Can you work these out from the model? Positions are in its coordinate system, mm. A direction names the side the tool comes from. Round coordinates to 2 decimals unless told otherwise and drop trailing zeros. Order: outer loops, then holes, each group sorted by start corner. A loop starts at its lowest first (then second) coordinate and runs counter-clockwise, first axis right, second up. Notation, with made-up numbers: M 39,-8 L 93,-8 A29 ccw 93,26 Z; hole C -13,-9.5 d4. An arc over 180 degrees is marked long. One line per question, with ' | ' between items.
```python
from build123d import *

# Parameters (mm, degrees)
SKETCH1_R           = 27.62
BOSS_EXTRUDE1_DEPTH = 6
SKETCH2_R           = 16
SKETCH2_R_2         = 14
BOSS_EXTRUDE2_DEPTH = 36
CUT_EXTRUDE1_START  = -36
SKETCH3_R           = 14
CUT_EXTRUDE1_DEPTH  = 36
CHAMFER1_SIZE       = 5
CHAMFER1_SIZE2      = 7.140740034
CHAMFER2_SIZE       = 1
SKETCH4_R           = 27
SKETCH4_R_2         = 25
CUT_EXTRUDE2_DEPTH  = 1.6
FILLET1_R           = 2
FILLET2_R           = 4


with BuildPart() as part:
    # Sketch1 → Boss-Extrude1 (new body)
    with BuildSketch(Plane(origin=(0, 0, 0), x_dir=(1, 0, 0), z_dir=(0, 1, 0))):
        with Locations(Location((0, 0, 0), (0, 0, 270))):
            Circle(SKETCH1_R)
    extrude(amount=BOSS_EXTRUDE1_DEPTH)

    # Sketch2 → Boss-Extrude2 (add)
    with BuildSketch(Plane(origin=(0, 6, 0), x_dir=(1, 0, 0), z_dir=(0, 1, 0))):
        with Locations(Location((0, 0, 0), (0, 0, 270))):
            Circle(SKETCH2_R)
        with Locations(Location((0, 0, 0), (0, 0, 270))):
            Circle(SKETCH2_R_2, mode=Mode.SUBTRACT)
    extrude(amount=BOSS_EXTRUDE2_DEPTH)

    # Sketch3 → Cut-Extrude1 (cut)
    with BuildSketch(Plane(origin=(0, 6, 0), x_dir=(1, 0, 0), z_dir=(0, 1, 0)).offset(CUT_EXTRUDE1_START)):
        with Locations(Location((0, 0, 0), (0, 0, 270))):
            Circle(SKETCH3_R)
    extrude(amount=CUT_EXTRUDE1_DEPTH, mode=Mode.SUBTRACT)

    # Chamfer1
    chamfer1_edges = [part.edges().sort_by_distance(p)[0] for p in [
        (0, 0, -14),
    ]]
    chamfer1_side = [part.faces().sort_by_distance(p)[0] for p in [
        (0, 21, -14),
    ]]
    chamfer(chamfer1_edges, length=CHAMFER1_SIZE, length2=CHAMFER1_SIZE2, reference=chamfer1_side[0])

    # Chamfer2
    chamfer2_edges = [part.edges().sort_by_distance(p)[0] for p in [
        (0, 6, -27.62),
    ]]
    chamfer(chamfer2_edges, length=CHAMFER2_SIZE)

    # Sketch4 → Cut-Extrude2 (cut)
    with BuildSketch(Plane.XZ):
        with Locations(Location((0, 0, 0), (0, 0, 270))):
            Circle(SKETCH4_R)
        with Locations(Location((0, 0, 0), (0, 0, 270))):
            Circle(SKETCH4_R_2, mode=Mode.SUBTRACT)
    extrude(amount=-CUT_EXTRUDE2_DEPTH, mode=Mode.SUBTRACT)

    # Fillet1
    fillet1_edges = [part.edges().sort_by_distance(p)[0] for p in [
        (0, 6, -16),
    ]]
    fillet(fillet1_edges, radius=FILLET1_R)

    # Fillet2
    fillet2_edges = [part.edges().sort_by_distance(p)[0] for p in [
        (0, 5, -14),
    ]]
    fillet(fillet2_edges, radius=FILLET2_R)


solid = part.part
```
(1) On a 3-axis mill with a long thin cutter (end or side, diameter ignored), from which of +Z, -Z, +X, -X, +Y, -Y can I reach the whole of each face in a straight line? I mean faces 4 (the cylindrical face through (7.509, 0.789, -23.846)), 5 (the flat face through (11, 0, -19)), 6 (the cylindrical face through (-15.62, 24.76, -3.47)). Say none if no direction works.
Final values:
face 4: -Y | face 5: +Z, -Z, +X, -X, -Y | face 6: +Y
(2) If we section it at A-A on y = 19.5: Please give me the cut outline in (x, z).
Final values:
outline: C 0,0 d32; hole C 0,0 d28
(3) Will these pins go through, and if not, where does the flat tip stop? pin 1 Ø12 at (x, y) = (-3.5, 20) entering from +Z; pin 2 Ø1 at (x, y) = (-3, 25) entering from -Z; pin 3 Ø2 at (x, y) = (7, 16.5) entering from +Z; pin 4 Ø3 at (x, z) = (-3.5, 16) entering from +Y.
Final values:
pin 1: z = 16 | pin 2: z = -15.8 | pin 3: z = 14.83 | pin 4: y = 42
(4) Thinking about a two-plate mould opening in Z: for faces 1 (the flat face through (-14.15, 42, -0.07)), 2 (the cylindrical face through (-5.362, 24.297, 12.932)), 3 (the cylindrical face through (-26.963, 2.465, -5.987)), which applies, released by +Z, released by -Z, zero draft, split by the parting line, or undercut?
Final values:
face 1: zero draft | face 2: undercut | face 3: split by the parting line
(5) Please list where these lines run through material, in increasing order: probe 1 along X at (y, z) = (16.5, 0); probe 2 along X at (y, z) = (0.65, 0); probe 3 along X at (y, z) = (1.3, 0). Write a range as [from, to].
Final values:
probe 1: [-16, -14], [14, 16] | probe 2: [-27.62, -27], [-25, -20.21], [20.21, 25], [27, 27.62] | probe 3: [-27.62, -27], [-25, -19.28], [19.28, 25], [27, 27.62]
